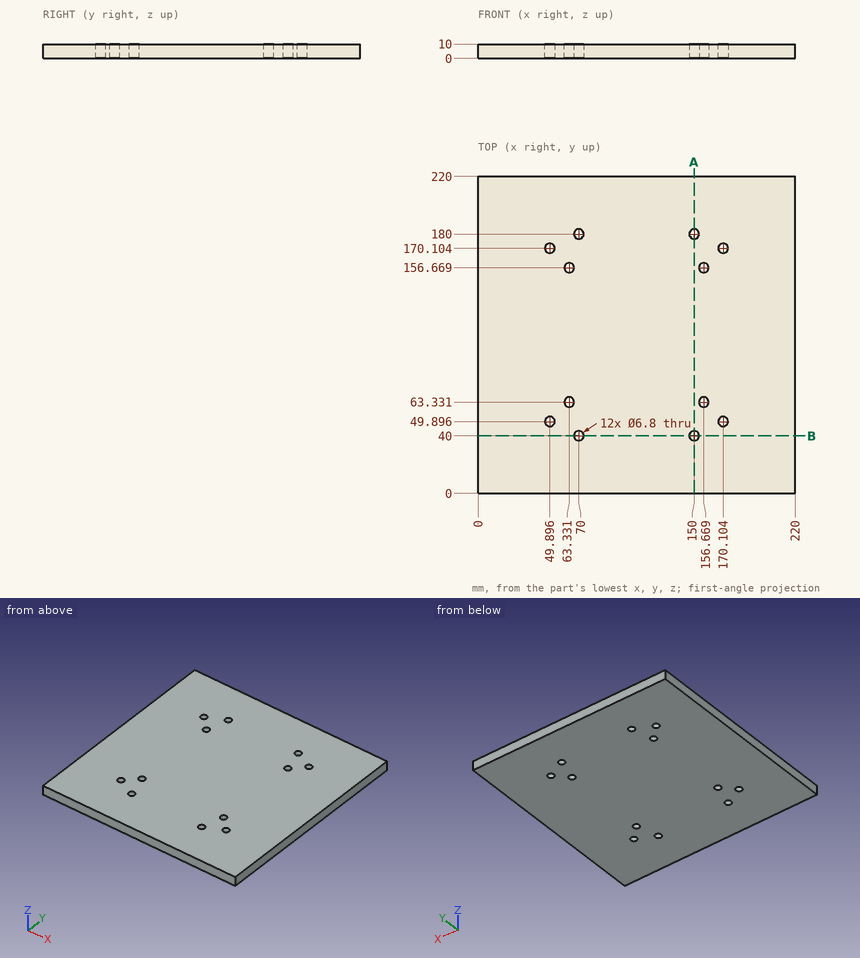
Job drawing, mm, ordinate dimensions from the low corner. One solid piece. Coordinates: 2 decimals unless noted, no trailing zeros. Write each loop counter-clockwise with the first axis right and the second up, starting at its lowest first coordinate (ties: lowest second). Pieces come first, ordered by that corner, then holes.
Item 1: Slice it at B-B (y = 40). Write the cut outline in (x, z), and give its area (3 significant figures).
Item 2: Slice it at A-A (x = 150). Write the cut outline in (y, z).
Item 3: Probe line 1 (X direction, y = 180, z = 5.5); line 2 (Y direction, x = 70, z = 6); line 3 (Y direction, x = 67.5, z = 3.5). List the from-to ranges inside material, lowest first.
Results found:
1. outline: (0, 0) - (66.6, 0) - (66.6, 10) - (0, 10) - close; (73.4, 0) - (146.6, 0) - (146.6, 10) - (73.4, 10) - close; (153.4, 0) - (220, 0) - (220, 10) - (153.4, 10) - close
1. area: 2,060 mm2
2. outline: (0, 0) - (36.6, 0) - (36.6, 10) - (0, 10) - close; (43.4, 0) - (176.6, 0) - (176.6, 10) - (43.4, 10) - close; (183.4, 0) - (220, 0) - (220, 10) - (183.4, 10) - close
3. line 1: x = 0 to 66.6, 73.4 to 146.6, 153.4 to 220
3. line 2: y = 0 to 36.6, 43.4 to 176.6, 183.4 to 220
3. line 3: y = 0 to 37.7, 42.3 to 177.7, 182.3 to 220
